```python
from build123d import *

# Parameters (mm, degrees)
SKETCH1_W           = 1
SKETCH1_H           = 1
BOSS_EXTRUDE1_DEPTH = 300
SKETCH2_W           = 1
SKETCH2_H           = 1
BOSS_EXTRUDE2_DEPTH = 100


with BuildPart() as part:
    # Sketch1 → Boss-Extrude1 (new body)
    with BuildSketch(Plane(origin=(0, 0, 0), x_dir=(0, 0, -1), z_dir=(1, 0, 0))):
        with Locations((0.137681159, -0.057971014)):
            Rectangle(SKETCH1_W, SKETCH1_H)
    extrude(amount=BOSS_EXTRUDE1_DEPTH)

    # Sketch2 → Boss-Extrude2 (add)
    with BuildSketch(Plane.XY.offset(0.362318841)):
        with Locations((199.5, -0.057971014)):
            Rectangle(SKETCH2_W, SKETCH2_H)
    extrude(amount=BOSS_EXTRUDE2_DEPTH)


solid = part.part
```
Read the model definition and answer for the solid it produces. Units are mm, in the model's axes. Round coordinates to 2 decimals unless told otherwise and drop trailing zeros. Write each loop counter-clockwise with the first axis right and the second up, starting at its lowest first coordinate (ties: lowest second). Pieces come first, ordered by that corner, then holes. Notation, with made-up numbers: M 12.25,42.25 L 40.25,42.25 A19 cw 40.25,72.25 Z; hole C 27,19.25 d3. An arc over 180 degrees is marked long. One line per item, written item: value.
Q1. Find section B-B on x = 72. Write down the section's boundary in (y, z), plus the area to 3 significant figures.
Data:
outline: M -0.56,-0.64 L 0.44,-0.64 L 0.44,0.36 L -0.56,0.36 Z
area: 1.00 mm2
Q2. Straight lines are drawn through the part: line 1 (Z direction, x = 201.5, y = 0.25); line 2 (X direction, y = 0.4, z = 15.5). For each, find the intervals that lie inside material, in ascending order. Write a range as [from, to].
Data:
line 1: [-0.64, 0.36]
line 2: [199, 200]
Q3. Find section A-A on y = 0.2. Write down the section's boundary in (x, z).
Data:
outline: M 0,-0.64 L 300,-0.64 L 300,0.36 L 200,0.36 L 200,100.36 L 199,100.36 L 199,0.36 L 0,0.36 Z
Q4. Find section C-C on z = 46.5. Write down the section's boundary in (x, y).
Data:
outline: M 199,-0.56 L 200,-0.56 L 200,0.44 L 199,0.44 Z
